Check sheet for the drawn part. Datum: minimum x, y, z corner. Units: mm. Coordinates: 2 decimals unless noted, no trailing zeros. Write each loop counter-clockwise with the first axis right and the second up, starting at its lowest first coordinate (ties: lowest second). Pieces come first, ordered by that corner, then holes. Notation, with made-up numbers: (-1.75, 33.25) - (57.25, 33.25) arc R10 cw to (57.25, 46.25) - close; hole circle Ø5 at (-25, 38.25). An arc over 180 degrees is marked (long way). Use one line per item in the form item = value. Start each with the question number.
1. Cross-section at C-C on x = 116.5. Record the boundary of the cut face in (y, z), then the cut area to 3 significant figures.
2. Scan line: line 1 along Z through (x, y) = (123, 62). Record every from-to range of solid material in increasing order.
3. Go/stop test with a flat-tipped pin: pin 1 Ø8 at (x, y) = (109, 59) entering from +Z. Record where the tip stops, or that it passes through.
4. Cross-section at A-A on y = 35. Record the boundary of the cut face in (x, z), then the cut area to 3 significant figures.
5. Cross-section at B-B on x = 15. Record the boundary of the cut face in (y, z), then the cut area to 3 significant figures.
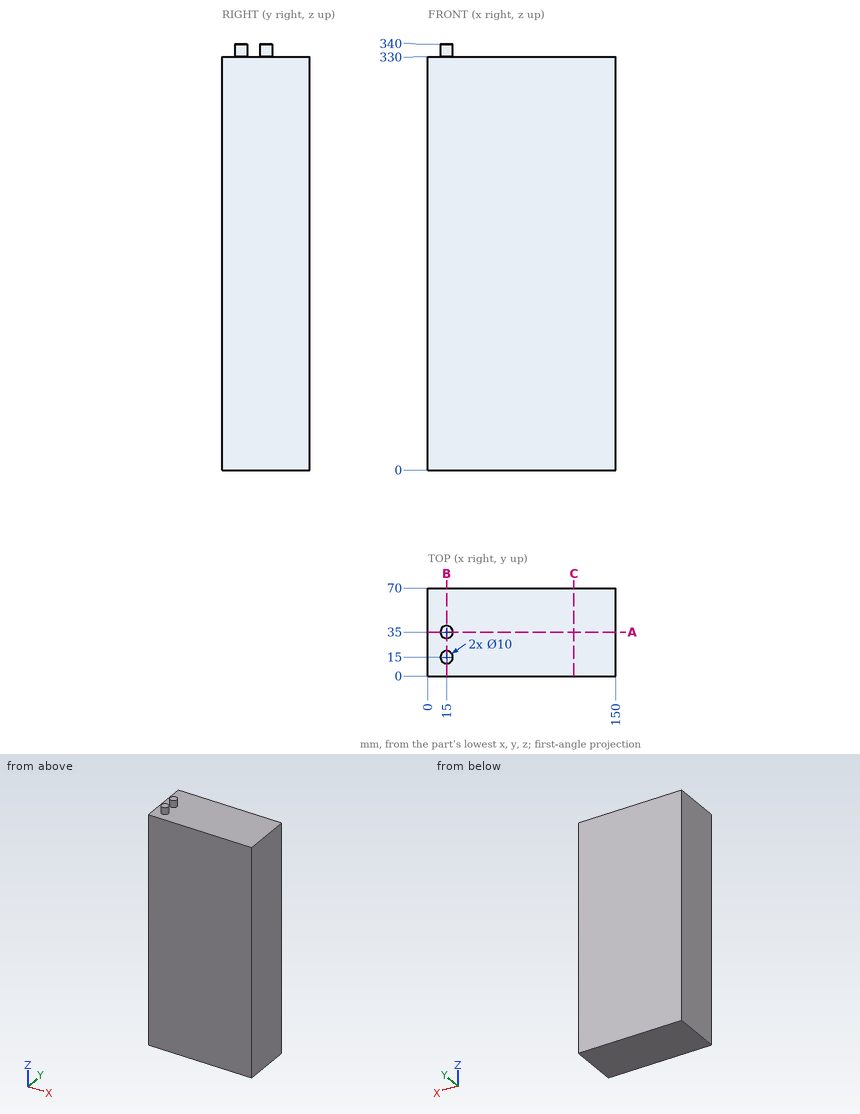
Final values:
q1.outline = (0, 0) - (70, 0) - (70, 330) - (0, 330) - close
q1.area = 23,100 mm²
q2.line_1 = 0 to 330
q3.pin_1 = 330
q4.outline = (0, 0) - (150, 0) - (150, 330) - (20, 330) - (20, 340) - (10, 340) - (10, 330) - (0, 330) - close
q4.area = 49,600 mm²
q5.outline = (0, 0) - (70, 0) - (70, 330) - (40, 330) - (40, 340) - (30, 340) - (30, 330) - (20, 330) - (20, 340) - (10, 340) - (10, 330) - (0, 330) - close
q5.area = 23,300 mm²
